```python
from build123d import *

# Parameters (mm, degrees)
F1_DEPTH = 12.7
F2_W     = 25.4
F2_H     = 12.7
F3_DEPTH = 38.1
F5_DEPTH = 12.7


# Not quite as in the source:
# - a feature names something its author has since deleted; it is built from what else it names


with BuildPart() as f1:
    # F0 (on Top) → F1 (new body)
    with BuildSketch(Plane.XY):
        Polygon((-9.6761901296, 0), (-47.7761901296, 0), (-47.7761901296, -12.7), (-22.3761901296, -12.7), align=None)
    extrude(amount=F1_DEPTH)

    # F2 (on Top) → F3 (join)
    with BuildSketch(Plane.XY):
        with Locations((-33.6697670078, 6.35)):
            Rectangle(F2_W, F2_H)
    extrude(amount=F3_DEPTH)

    # F4 (on Front) → F5 (join)
    with BuildSketch(Plane.XZ):
        Polygon((-21.0471171886, 37.6062467694), (-21.3566347957, 0), (-8.9759770781, 0), (-8.9759770781, 14.0829980373), align=None)
    extrude(amount=-F5_DEPTH)


solid = f1.part
```
Can you work these out from the model? Positions are in its coordinate system, mm. A direction names the side the tool comes from. Give positions to 0.01 mm unless a question says otherwise; leave off trailing zeros. Loops run counter-clockwise (first coordinate to the right, second up) from the corner with the lowest first, then second, coordinate; pieces in that order, holes last. Notation, with made-up numbers: M -22,45.5 L 9,45.5 A20 cw 9,84.5 Z; hole C -38.5,-36.75 d10. An arc over 180 degrees is marked long. Use CSV: the item, a comma, the result in double quotes. Start each with the question number.
1. Imagine slicing it at D-D, the plane z = 20. Write out the boundary of the cut face in (x, y), plus the area to 3 significant figures.
2. Imagine slicing it at A-A, the plane z = 11.5. Write out the boundary of the cut face in (x, y).
3. If I drill on L1, parallel to Z at x = -30, y = -1; L2, parallel to X at y = 4, z = 9, over which ranges is the centre line in solid material (lowest first)?
4. Imagine slicing it at B-B, the plane x = -25.5. Write out the boundary of the cut face in (y, z), plus the area to 3 significant figures.
5. For P1, Ø0.5, axis at y = 7.5, z = 38, coming from the +X side; P2, Ø2, axis at y = -1.5, z = 6.5, coming from the +X side; P3, Ø6.5, axis at y = 8, z = 16, coming from the -X side; P4, Ø5, axis at y = -3.5, z = 29, coming from the -X side, each with a flat end and sliding along its axis, tell me the tip position at first contact or that it passes through.
6. Imagine slicing it at C-C, the plane y = 0.5. Write out the boundary of the cut face in (x, z).
7. On a 3-axis mill with a long thin cutter (end or side, diameter ignored), from which of +Z, -Z, +X, -X, +Y, -Y can I reach the whole of each face in a straight line? I mean faces 1 (the face through (-29, 0, 0)), 2 (the face through (-33, -6, 12.7)), 3 (the face through (-46.37, 6, 19)). Say none if no direction works.
Response values:
1,outline,"M -46.37,0 L -12.01,0 L -12.01,12.7 L -46.37,12.7 Z"
1,area,"436 mm^2"
2,outline,"M -47.78,-12.7 L -22.38,-12.7 L -9.68,0 L -8.98,0 L -8.98,12.7 L -46.37,12.7 L -46.37,0 L -47.78,0 Z"
3,L1,"0 to 12.7"
3,L2,"-46.37 to -8.98"
4,outline,"M -12.7,0 L 12.7,0 L 12.7,38.1 L 0,38.1 L 0,12.7 L -12.7,12.7 Z"
4,area,"645 mm^2"
5,P1,"x = -20.97"
5,P2,"x = -10.18"
5,P3,"x = -46.37"
5,P4,"through"
6,outline,"M -46.37,0 L -8.98,0 L -8.98,14.08 L -20.97,37.46 L -20.97,38.1 L -46.37,38.1 Z"
7,face 1,"-Z, +X, -X, +Y, -Y"
7,face 2,"+Z, +X, -X, -Y"
7,face 3,"+Z, -Z, -X, +Y"
